Source: CAD feature listing. Evaluate the final solid. Frame: model axes, mm. A direction names the side the tool comes from. Give positions to 0.01 mm unless a question says otherwise; leave off trailing zeros. Loops run counter-clockwise (first coordinate to the right, second up) from the corner with the lowest first, then second, coordinate; pieces in that order, holes last.
```python
from build123d import *

# Parameters (mm, degrees)
SKETCH1_W           = 160
SKETCH1_H           = 15
BOSS_EXTRUDE1_DEPTH = 4
BOSS_EXTRUDE2_DEPTH = 4


with BuildPart() as part:
    # Sketch1 → Boss-Extrude1 (new body)
    with BuildSketch(Plane(origin=(0, 0, 0), x_dir=(1, 0, 0), z_dir=(0, 1, 0))):
        with Locations((-45.993031359, 57.116724739)):
            Rectangle(SKETCH1_W, SKETCH1_H)
    extrude(amount=BOSS_EXTRUDE1_DEPTH)

    # Sketch2 → Boss-Extrude2 (add)
    with BuildSketch(Plane(origin=(0, 0, 0), x_dir=(1, 0, 0), z_dir=(0, 1, 0))):
        Polygon((-125.993031359, 64.616724739), (-25.993031359, 64.616724739), (34.006968641, 69.116724739), (34.006968641, 45.116724739), (-25.993031359, 49.616724739), (-125.993031359, 49.616724739), align=None)
    extrude(amount=-BOSS_EXTRUDE2_DEPTH)


solid = part.part
```
(1) Ray query, line 1 along Z through (x, y) = (-60, -2); line 2 along Z through (x, y) = (-6.5, -2). Return the intervals inside material, ascending.
A:
line 1: z = -64.62 to -49.62
line 2: z = -66.08 to -48.15
(2) First-contact query: pin 1 (3 mm diameter, centred on x = -73.5, y = -0.5, fed in from +Z); pin 2 (2 mm diameter, centred on x = -51, y = -1, fed in from -Z); pin 3 (3.5 mm diameter, centred on x = 7, z = -47, fed in from +Y). Flat tips, straight axial feed; report the tip coordinate or a pass-through.
A:
pin 1: stops at z = -49.62
pin 2: stops at z = -64.62
pin 3: stops at y = 0
(3) Section D-D, the plane x = -91. Return the cut outline in (y, z).
A:
outline: (-4, -64.62) - (4, -64.62) - (4, -49.62) - (-4, -49.62) - close
(4) Section B-B, the plane x = 18. Return the cut outline in (y, z), then the cut area to 3 significant figures.
A:
outline: (-4, -67.92) - (0, -67.92) - (0, -64.62) - (4, -64.62) - (4, -49.62) - (0, -49.62) - (0, -46.32) - (-4, -46.32) - close
area: 146 mm2
(5) Reachability of faces 1 (the flat face through (-63, 0, -49.617)), 2 (the flat face through (18, 0, -66)), 3 (the flat face through (11, 0, -48)), 4 (the flat face through (-65, 0, -64.617)), 5 (the flat face through (-45, -4, -57)) from +Z, -Z, +X, -X, +Y, -Y: full face, straight path, thin tool, end or side. Return the list, or none.
A:
face 1: +Z, -X, +Y
face 2: -Z, +X, -X, +Y
face 3: +Z, +X, -X, +Y
face 4: -Z, -X, +Y
face 5: +Z, -Z, +X, -X, -Y
(6) Section C-C, the plane z = -67.5. Return the cut outline in (x, y).
A:
outline: (12.45, -4) - (34.01, -4) - (34.01, 0) - (12.45, 0) - close
(7) Mould query, pull axis Z, two halves, no side actions, for faces 6 (the flat face through (4.427, -1.972, -47.335)), 7 (the flat face through (3.587, -1.972, -66.835)), 8 (the flat face through (-125.993, 0, -57)). Classes: pulls with the +Z half, pulls with the -Z half, needs draft (parallel to the pull), parting line crosses it, or undercut.
A:
face 6: pulls with the +Z half
face 7: pulls with the -Z half
face 8: needs draft
(8) Section A-A, the plane y = -2.75. Return the cut outline in (x, z), then the cut area to 3 significant figures.
A:
outline: (-125.99, -64.62) - (-25.99, -64.62) - (34.01, -69.12) - (34.01, -45.12) - (-25.99, -49.62) - (-125.99, -49.62) - close
area: 2,670 mm2
